Geometry: final body of the model. Coordinates: model frame, mm. A direction names the side the tool comes from. Give positions to 0.01 mm unless a question says otherwise; leave off trailing zeros. Write each loop counter-clockwise with the first axis right and the second up, starting at its lowest first coordinate (ties: lowest second). Pieces come first, ordered by that corner, then holes. Notation, with made-up numbers: (59, 55.5) - (99, 55.5) arc R8 cw to (99, 61.5) - close; hole circle Ø9 at (21, 54.5). An arc over 180 degrees is marked (long way). One line per question, with ' | ' between items. Start each with the question number.
```python
from build123d import *

# Parameters (mm, degrees)
PAD_DEPTH       = 20
POCKET_DEPTH    = 5
POCKET001_DEPTH = 5
PAD001_DEPTH    = 2.5
SKETCH004_W     = 1.549321
SKETCH004_H     = 7.389076
POCKET002_DEPTH = 20.001
POCKET003_DEPTH = 20.001
POCKET004_DEPTH = 20.001
POCKET005_DEPTH = 20.001


with BuildPart() as part:
    # Sketch → Pad (new body)
    with BuildSketch(Plane.XY):
        Polygon((-9.801471, 25.959593), (11.01361, 25.959593), (20.613062, 9.803649), (10.505054, 0), (10.505054, -10.208122), (-10.014578, -10.208122), (-10.216599, 0), (-20.202017, 10.202021), align=None)
    extrude(amount=PAD_DEPTH)

    # Sketch002 (on Face10 of Pad) → Pocket (cut)
    with BuildSketch(Plane.XY.offset(20)):
        Polygon((10.707072, 10.808081), (3.03031, 10.808081), (6.868694, 17.474747), align=None)
    extrude(amount=-POCKET_DEPTH, mode=Mode.SUBTRACT)

    # Sketch001 (on Face10 of Pad) → Pocket001 (cut)
    with BuildSketch(Plane.XY.offset(20)):
        Polygon((-6.060602, 16.262627), (-9.696968, 10.606062), (-3.030296, 10.606062), align=None)
    extrude(amount=-POCKET001_DEPTH, mode=Mode.SUBTRACT)

    # Sketch003 (on Face5 of Pocket001) → Pad001 (join)
    with BuildSketch(Plane.XY.offset(20)):
        Polygon((0, 7.979798), (-3.030296, 3.535354), (2.424244, 2.929294), align=None)
    extrude(amount=PAD001_DEPTH)

    # Sketch004 (on Face5 of Pad001) → Pocket002 (cut, through all)
    with BuildSketch(Plane.XY.offset(20)):
        with Locations((-6.289715, -4.81679)):
            Rectangle(SKETCH004_W, SKETCH004_H)
    extrude(amount=-POCKET002_DEPTH, mode=Mode.SUBTRACT)

    # Sketch005 (on Face5 of Pocket002) → Pocket003 (cut, through all)
    with BuildSketch(Plane.XY.offset(20)):
        Polygon((-2.178051, -1.718145), (-2.178051, -8.749685), (0, -8.511328), (-0.032834, -1.718145), align=None)
    extrude(amount=-POCKET003_DEPTH, mode=Mode.SUBTRACT)

    # Sketch006 (on Face5 of Pocket003) → Pocket004 (cut, through all)
    with BuildSketch(Plane.XY.offset(20)):
        Polygon((1.874023, -1.36061), (1.754846, -8.749685), (4.019244, -9.226399), (3.661705, -1.241431), align=None)
    extrude(amount=-POCKET004_DEPTH, mode=Mode.SUBTRACT)

    # Sketch007 (on Face5 of Pocket004) → Pocket005 (cut, through all)
    with BuildSketch(Plane.XY.offset(20)):
        Polygon((5.449386, -1.718145), (5.926099, -9.345578), (7.475415, -8.630507), (7.475415, -1.598966), align=None)
    extrude(amount=-POCKET005_DEPTH, mode=Mode.SUBTRACT)


solid = part.part
```
1) Section C-C, the plane z = 17.5. Give the number of separate pieces and of enclosed holes in the cut face, plus the area to 3 significant figures.
2) Pull-direction query (X, two-part tool) for faces 1 (the flat face through (-15.075, 17.971, 9.86)), 2 (the flat face through (-6, -1.122, 10)), 3 (the flat face through (15.75, 17.99, 9.86)); classes: +X half, -X half, draft (parallel to the pull), parting line (faces both ways), or undercut.
3) Section B-B, the plane x = -1.5. Output: boundary loops of the cut face in (y, z).
4) Section A-A, the plane z = 4.75. Output: boundary loops of the cut face in (x, y), plus the area to 3 significant figures.
5) Reachability of faces 4 (the flat face through (-4.52, 13.39, 17.54)), 5 (the flat face through (-6, -8.511, 10)), 6 (the flat face through (-1.494, 5.789, 21.232)), 7 (the flat face through (10.505, -5, 10)), 8 (the flat face through (1.23, 5.42, 21.23)) from +Z, -Z, +X, -X, +Y, -Y: full face, straight path, thin tool, end or side. Return the list, or none.
6) Section D-D, the plane y = 12. Output: boundary loops of the cut face in (x, z).
7) Line query: L1, parallel to Z at x = -8.5, y = 6; L2, parallel to X at y = -6.5, z = 14.75; L3, parallel to Y at x = 3, z = 3. Output: solid intervals per line, ascending.
8) First-contact query: pin 1 Ø5 at (y, z) = (-4, 6) entering from +X; pin 2 Ø3 at (x, z) = (13, 10.5) entering from +Y; pin 3 Ø1 at (x, y) = (-9, 6) entering from +Z. Flat tips, straight axial feed; report the tip coordinate or a pass-through.
Answer key:
1) separate pieces: 1 | enclosed holes: 6 | area: 910 mm^2
2) face 1: -X half | face 2: undercut | face 3: +X half
3) outline: (-10.21, 0) - (-8.68, 0) - (-8.68, 20) - (-10.21, 20) - close; (-1.72, 0) - (25.96, 0) - (25.96, 20) - (5.78, 20) - (5.78, 22.5) - (3.37, 22.5) - (3.37, 20) - (-1.72, 20) - close
4) outline: (-20.2, 10.2) - (-10.22, 0) - (-10.01, -10.21) - (10.51, -10.21) - (10.51, 0) - (20.61, 9.8) - (11.01, 25.96) - (-9.8, 25.96) - close; hole (-7.06, -8.51) - (-5.52, -8.51) - (-5.52, -1.12) - (-7.06, -1.12) - close; hole (-2.18, -8.75) - (0, -8.51) - (-0.03, -1.72) - (-2.18, -1.72) - close; hole (1.75, -8.75) - (4.02, -9.23) - (3.66, -1.24) - (1.87, -1.36) - close; hole (5.45, -1.72) - (5.93, -9.35) - (7.48, -8.63) - (7.48, -1.6) - close | area: 955 mm^2
5) face 4: +Z | face 5: +Z, -Z | face 6: +Z, -X, +Y | face 7: +Z, -Z, +X, -Y | face 8: +Z, +X, +Y
6) outline: (-19.02, 0) - (19.31, 0) - (19.31, 20) - (10.02, 20) - (10.02, 15) - (3.72, 15) - (3.72, 20) - (-3.78, 20) - (-3.78, 15) - (-8.8, 15) - (-8.8, 20) - (-19.02, 20) - close
7) L1: 0 to 20 | L2: -10.09 to -7.06, -5.52 to -2.18, -0.01 to 1.79, 3.9 to 5.75, 7.48 to 10.51 | L3: -10.21 to -9.01, -1.29 to 25.96
8) pin 1: x = 10.51 | pin 2: y = 25.14 | pin 3: z = 20
